from build123d import *

# Parameters (mm, degrees)
F1_DEPTH       = 20
F2_R           = 9.99999
F4_D           = 13.2
F4_CBORE_D     = 19.25
F4_CBORE_DEPTH = 0


# Not quite as in the source:
# - a fillet or chamfer is up to 0.001 mm smaller than in the source, because OpenCascade refuses the exact size


with BuildPart() as f1:
    # F0 (on Front) → F1 (new body)
    with BuildSketch(Plane.XZ):
        Polygon((46.0956162758, 6.5648934066), (-18.9043837242, 6.5648934066), (-18.9043837242, -13.4351065934), (6.0956162758, -13.4351065934), (21.0956162758, -32.5433855138), (46.0956162758, -32.5433855138), align=None)
    extrude(amount=F1_DEPTH)

    # F2 (radius 10 in the source; OpenCascade refuses exactly that, so slightly less here)
    f2_edges = [f1.edges().sort_by_distance(p)[0] for p in [
        (-18.904384, 0, -3.435107),
        (-18.904384, -20, -3.435107),
    ]]
    fillet(f2_edges, radius=F2_R)

    # F4 (through all)
    with Locations(Plane.XY.offset(6.5648934066)):
        with Locations((-8.9043837242, -10), (36.0956162758, -10)):
            CounterBoreHole(F4_D / 2, F4_CBORE_D / 2, F4_CBORE_DEPTH)


solid = f1.part
Part model, mm, in its own coordinate system. A direction names the side the tool comes from. Coordinates: 2 decimals unless noted, no trailing zeros. Order: outer loops, then holes, each group sorted by start corner. A loop starts at its lowest first (then second) coordinate and runs counter-clockwise, first axis right, second up. Notation, with made-up numbers: M -36.5,54 L -6.5,54 A19 cw -6.5,66 Z; hole C 0,32 d10. An arc over 180 degrees is marked long. One line per question, with ' | ' between items.
Q1. Pin check, flat tips, straight feed: P1, Ø10, axis at x = -7.5, y = -18, coming from the -Z side; P2, Ø12, axis at x = 36.1, y = -10, coming from the +Z side; P3, Ø3, axis at y = -3.5, z = -8.5, coming from the -X side; P4, Ø5, axis at y = -16.5, z = -14, coming from the -X side. Stop position of each tip, or through.
A:
P1: stops at z = -13.44 | P2: passes through | P3: stops at x = -17.56 | P4: stops at x = -18.04
Q2. Slice it at B-B (y = -5). Give the cut face in (x, z).
A:
outline: M -17.56,-13.44 L -13.21,-13.44 L -13.21,6.56 L -17.56,6.56 Z; M -4.6,-13.44 L 6.1,-13.44 L 21.1,-32.54 L 31.79,-32.54 L 31.79,6.56 L -4.6,6.56 Z; M 40.4,-32.54 L 46.1,-32.54 L 46.1,6.56 L 40.4,6.56 Z
Q3. Slice it at C-C (x = -3.5). Give the cut face in (y, z).
A:
outline: M -20,-13.44 L -13.79,-13.44 L -13.79,6.56 L -20,6.56 Z; M -6.21,-13.44 L 0,-13.44 L 0,6.56 L -6.21,6.56 Z
Q4. Drill centre lines: line 1 (X direction, y = -10.75, z = -12); line 2 (X direction, y = -9, z = -13); line 3 (Y direction, x = -9, z = -8.5). Where is each one in solid material? Low to high.
A:
line 1: x = -18.88 to -15.46, -2.35 to 29.54, 42.65 to 46.1 | line 2: x = -18.85 to -15.43, -2.38 to 29.57, 42.62 to 46.1 | line 3: y = -20 to -16.6, -3.4 to 0
Q5. Slice it at A-A (z = 4.5). Count the separate pieces of the cut face and the enclosed holes in it, and give its area (3 significant figures).
A:
separate pieces: 1 | enclosed holes: 2 | area: 983 mm^2
Q6. Two-plate mould, pull along X, no slides. Class faces 3 (the face through (-16.053, -3.007, -3.575)), 4 (the face through (24, 0, -8)), 5 (the face through (29.8, -8.02, -13.26)), 6 (the face through (-15.2, -8.02, -3.58)): +X half, -X half, draft (parallel to the pull), parting line (faces both ways), or undercut.
A:
face 3: -X half | face 4: draft | face 5: undercut | face 6: undercut
Q7. 3-axis set-ups, long thin cutter, end or side, ignore diameter. For faces 1 (the face through (-1, -10, -13.435)), 2 (the face through (24, -20, -8)): which of +Z, -Z, +X, -X, +Y, -Y reach the whole face in a straight line?
A:
face 1: -Z, -X, +Y, -Y | face 2: +Z, -Z, +X, -X, -Y
Q8. Slice it at D-D (z = -25.5). Give the cut face in (x, y).
A:
outline: M 15.57,-20 L 46.1,-20 L 46.1,0 L 15.57,0 Z; hole C 36.1,-10 d13.2
